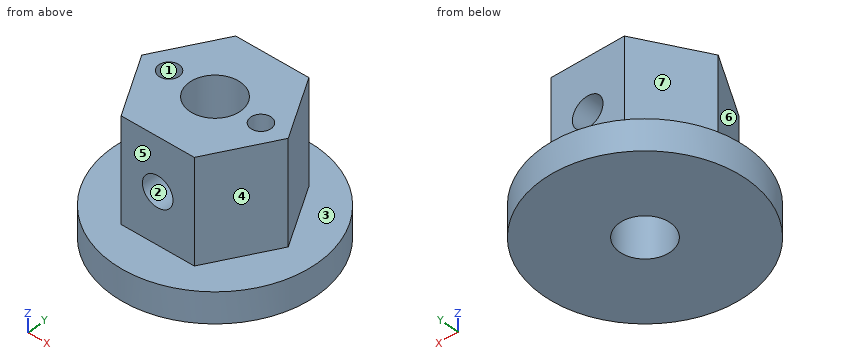
```python
from build123d import *

# Parameters (mm, degrees)
SKETCH_R      = 2.5
SKETCH_R_2    = 1
PAD_DEPTH     = 10.15
SKETCH001_R   = 1.5
POCKET_DEPTH  = 12.419804
SKETCH002_R   = 10
SKETCH002_R_2 = 2.5
PAD001_DEPTH  = 3


with BuildPart() as part:
    # Sketch → Pad (new body)
    with BuildSketch(Plane.XY):
        Polygon((-7.17, 0), (-3.585, -6.209402), (3.585, -6.209402), (7.17, 0), (3.585, 6.209402), (-3.585, 6.209402), align=None)
        Circle(SKETCH_R, mode=Mode.SUBTRACT)
        with Locations((4.5, 0)):
            Circle(SKETCH_R_2, mode=Mode.SUBTRACT)
        with Locations((-4.5, 0)):
            Circle(SKETCH_R_2, mode=Mode.SUBTRACT)
    extrude(amount=PAD_DEPTH)

    # Sketch001 → Pocket (cut, through all)
    with BuildSketch(Plane(origin=(0, 6.209402, 0), x_dir=(-1, 0, 0), z_dir=(0, 1, 0))):
        with Locations((0, 5)):
            Circle(SKETCH001_R)
    extrude(amount=-POCKET_DEPTH, mode=Mode.SUBTRACT)

    # Sketch002 → Pad001 (new body)
    with BuildSketch(Plane(origin=(0, 0, 0), x_dir=(1, 0, 0), z_dir=(0, 0, -1))):
        Circle(SKETCH002_R)
        Circle(SKETCH002_R_2, mode=Mode.SUBTRACT)
    extrude(amount=PAD001_DEPTH)


solid = part.part
```
Verification items for the finished model (mm, model axes). Face numbers are marked on the shaded views. A direction names the side the tool comes from. Give positions to 0.01 mm unless a question says otherwise; leave off trailing zeros. Order: outer loops, then holes, each group sorted by start corner. A loop starts at its lowest first (then second) coordinate and runs counter-clockwise, first axis right, second up. Notation, with made-up numbers: (89, 68.25) -> (126, 68.25) arc R11 ccw to (126, 78.25) -> close; hole circle Ø9 at (50.25, -20.5). An arc over 180 degrees is marked (long way). Use a Markdown table: item, result.
1) Section check D-D, the plane y = 4.25. Record the boundary of the cut face in (x, z), then the cut area to 3 significant figures.
Results:
| item | result |
|---|---|
| outline | (-9.05, -3) -> (9.05, -3) -> (9.05, 0) -> (4.72, 0) -> (4.72, 10.15) -> (-4.72, 10.15) -> (-4.72, 0) -> (-9.05, 0) -> close; hole circle Ø3 at (0, 5) |
| area | 143 mm² |
2) Depth check by flat-ended pin: pin 1 Ø3.5 at (x, z) = (1, 7) entering from -Y; pin 2 Ø1.8 at (x, y) = (-4.5, 0) entering from +Z; pin 3 Ø4 at (y, z) = (6, 6.5) entering from +X. Enter the tip coordinate at first touch or a pass-through.
Results:
| item | result |
|---|---|
| pin 1 | y = -6.21 |
| pin 2 | z = 0 |
| pin 3 | x = 4.86 |
3) Mould release check, pull along Z, two halves, no side actions. Record for the marked faces 1, 2 and 3: pulls with the +Z half, pulls with the -Z half, needs draft (parallel to the pull), parting line crosses it, or undercut.
Results:
| item | result |
|---|---|
| face 1 | needs draft |
| face 2 | undercut |
| face 3 | pulls with the +Z half |
4) Section check C-C, the plane z = 4. Record the boundary of the cut face in (x, y) (3 decimals), then the cut area to 3 significant figures.
Results:
| item | result |
|---|---|
| outline | (-7.17, 0) -> (-3.585, -6.209) -> (-1.118, -6.209) -> (-1.118, -2.236) arc R2.5 cw to (-1.118, 2.236) -> (-1.118, 6.209) -> (-3.585, 6.209) -> close; (1.118, -6.209) -> (3.585, -6.209) -> (7.17, 0) -> (3.585, 6.209) -> (1.118, 6.209) -> (1.118, 2.236) arc R2.5 cw to (1.118, -2.236) -> close; hole circle Ø2 at (-4.5, 0); hole circle Ø2 at (4.5, 0) |
| area | 90.7 mm² |
5) Tool access check on the marked faces 4, 5, 6 and 7. Record the directions out of +Z, -Z, +X, -X, +Y, -Y that give a thin tool (end or side, any length) a straight path to the whole face; none if there is none.
Results:
| item | result |
|---|---|
| face 4 | +Z, +X, -Y |
| face 5 | +Z, +X, -X, -Y |
| face 6 | +Z, -X, -Y |
| face 7 | +Z, -X, +Y |
6) Material ranges on probe 1 along Z at (x, y) = (0, 3.55); probe 2 along Y at (x, z) = (1.5, 5.5); probe 3 along X at (y, z) = (1.5, 6), recorded low to high.
Results:
| item | result |
|---|---|
| probe 1 | -3 to 3.5, 6.5 to 10.15 |
| probe 2 | -6.21 to -2, 2 to 6.21 |
| probe 3 | -6.3 to -2, 2 to 6.3 |
7) Section check A-A, the plane z = 0.25. Record the boundary of the cut face in (x, y) (3 decimals), then the cut area to 3 significant figures.
Results:
| item | result |
|---|---|
| outline | (-7.17, 0) -> (-3.585, -6.209) -> (3.585, -6.209) -> (7.17, 0) -> (3.585, 6.209) -> (-3.585, 6.209) -> close; hole circle Ø2 at (-4.5, 0); hole circle Ø5 at (0, 0); hole circle Ø2 at (4.5, 0) |
| area | 108 mm² |
8) Section check B-B, the plane x = 0. Record the boundary of the cut face in (y, z).
Results:
| item | result |
|---|---|
| outline | (-10, -3) -> (-2.5, -3) -> (-2.5, 3.5) -> (-6.21, 3.5) -> (-6.21, 0) -> (-10, 0) -> close; (-6.21, 6.5) -> (-2.5, 6.5) -> (-2.5, 10.15) -> (-6.21, 10.15) -> close; (2.5, -3) -> (10, -3) -> (10, 0) -> (6.21, 0) -> (6.21, 3.5) -> (2.5, 3.5) -> close; (2.5, 6.5) -> (6.21, 6.5) -> (6.21, 10.15) -> (2.5, 10.15) -> close |
